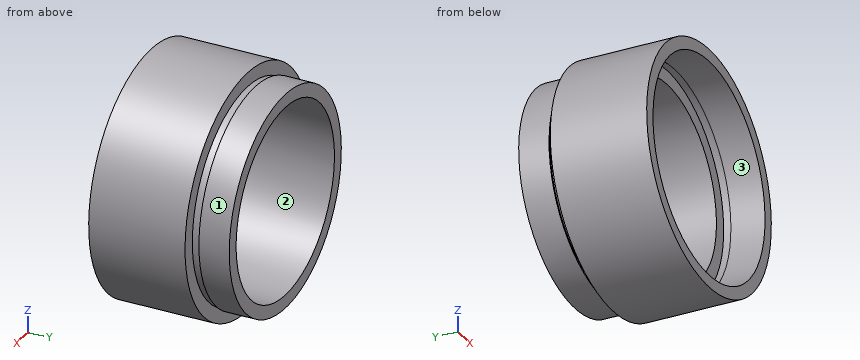
from build123d import *


with BuildPart() as part:
    # 草图1 → 旋转1 (revolve)
    with BuildSketch(Plane.XY, mode=Mode.PRIVATE) as revolve_1_sk:
        Polygon((14.25, 0), (14.25, 4.5), (14.35, 4.5), (14.35, 5.5), (12.5, 5.5), (12.5, 17.7), (14.25, 17.7), (14.25, 13.7), (14, 13.7), (14, 12.7), (15.85, 12.7), (15.85, 0), align=None)
    revolve(revolve_1_sk.sketch.rotate(Axis((0, 161.376166943, 0), (0, -1, 0)), 90), axis=Axis((0, 161.376166943, 0), (0, -1, 0)))  # turned: the seam where the file's is


solid = part.part
Source: CAD feature listing. Evaluate the final solid. Frame: model axes, mm. Face numbers are marked on the shaded views. Coordinates: 2 decimals unless noted, no trailing zeros. Order: outer loops, then holes, each group sorted by start corner. A loop starts at its lowest first (then second) coordinate and runs counter-clockwise, first axis right, second up.
Item 1: Pull-direction query (X, two-part tool) for the marked faces 1, 2 and 3; classes: pulls with the +X half, pulls with the -X half, needs draft (parallel to the pull), parting line crosses it, or undercut.
Output values:
face 1: parting line crosses it
face 2: undercut
face 3: undercut
Item 2: Cut plane B-B (x = 0). Return loops of the section in (y, z), plus the area to 3 significant figures.
Output values:
outline: (0, -15.85) - (12.7, -15.85) - (12.7, -14) - (13.7, -14) - (13.7, -14.25) - (17.7, -14.25) - (17.7, -12.5) - (5.5, -12.5) - (5.5, -14.35) - (4.5, -14.35) - (4.5, -14.25) - (0, -14.25) - close; (0, 14.25) - (4.5, 14.25) - (4.5, 14.35) - (5.5, 14.35) - (5.5, 12.5) - (17.7, 12.5) - (17.7, 14.25) - (13.7, 14.25) - (13.7, 14) - (12.7, 14) - (12.7, 15.85) - (0, 15.85) - close
area: 82.6 mm2
Item 3: Cut plane D-D (y = 14.75). Return loops of the section in (x, z).
Output values:
outline: circle Ø28.5 at (0, 0); hole circle Ø25 at (0, 0)
Item 4: First-contact query: P1, Ø6, axis at x = -4.5, y = 12.5, coming from the +Z side; P2, Ø8, axis at x = -9.5, z = -1, coming from the -Y side; P3, Ø3, axis at y = 6, z = 11.5, coming from the -X side. Flat tips, straight axial feed; report the tip coordinate or a pass-through.
Output values:
P1: stops at z = 15.78
P2: stops at y = 5.5
P3: stops at x = -12.3
Item 5: Material intervals for line 1 (X direction, y = 2.8, z = 0); line 2 (X direction, y = 16.5, z = 0); line 3 (Z direction, x = 0.5, y = 2.5), sorted ascending.
Output values:
line 1: x = -15.85 to -14.25, 14.25 to 15.85
line 2: x = -14.25 to -12.5, 12.5 to 14.25
line 3: z = -15.84 to -14.24, 14.24 to 15.84
Item 6: Cut plane C-C (y = 9). Return loops of the section in (x, z), plus the area to 3 significant figures.
Output values:
outline: circle Ø31.7 at (0, 0); hole circle Ø25 at (0, 0)
area: 298 mm2
Item 7: Cut plane A-A (z = 0). Return loops of the section in (x, y).
Output values:
outline: (-15.85, 0) - (-14.25, 0) - (-14.25, 4.5) - (-14.35, 4.5) - (-14.35, 5.5) - (-12.5, 5.5) - (-12.5, 17.7) - (-14.25, 17.7) - (-14.25, 13.7) - (-14, 13.7) - (-14, 12.7) - (-15.85, 12.7) - close; (12.5, 5.5) - (14.35, 5.5) - (14.35, 4.5) - (14.25, 4.5) - (14.25, 0) - (15.85, 0) - (15.85, 12.7) - (14, 12.7) - (14, 13.7) - (14.25, 13.7) - (14.25, 17.7) - (12.5, 17.7) - close
